Here's how the part is built. I have some questions about the finished solid (model axes, mm). Round coordinates to 2 decimals unless told otherwise and drop trailing zeros. Order: outer loops, then holes, each group sorted by start corner. A loop starts at its lowest first (then second) coordinate and runs counter-clockwise, first axis right, second up. Notation, with made-up numbers: (-0.75, -22.75) - (31.25, -22.75) arc R17 ccw to (31.25, -16.75) - close; hole circle Ø9 at (43, 6.25). An arc over 180 degrees is marked (long way). One line per item, written item: value.
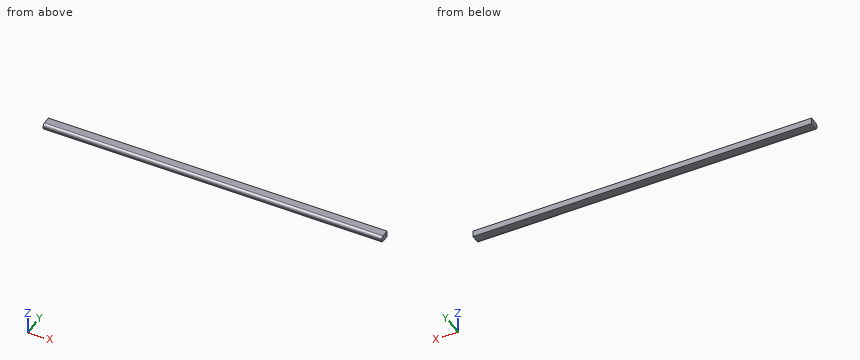
Autodesk Inventor part; units mm, degrees
ref_plane "YZ Plane" through (0, 0, 0) normal (1, 0, 0) x (0, 1, 0)
ref_plane "XZ Plane" through (0, 0, 0) normal (0, 1, 0) x (-1, 0, 0)
ref_plane "XY Plane" through (0, 0, 0) normal (0, 0, 1) x (1, 0, 0)
sketch "Sketch1" plane through (0, 0, 0) normal (0, 0, 1) x (1, 0, 0)
  line L0 (-592, 18) -> (592, 18)
  line L1 (592, 18) -> (592, -18)
  line L2 (592, -18) -> (-592, -18)
  line L3 (-592, -18) -> (-592, 18)
  line L4 (-592, 18) -> (592, -18) construction
  line L5 (592, 18) -> (-592, -18) construction
  point P0 (0, 0)
  dimension "d0" = 36
  dimension "d1" = 1184
extrude "Extrusion1" add sketch "Sketch1" along normal blind 22
fillet "Fillet1" radius 10 1 edges at (0, -18, 22)
fillet "Fillet2" radius 10 1 edges at (0, -18, 0)
properties part number "Light tube 118.4cm"
Q1. Will these pins go through, and if not, where does the flat tip stop? pin 1 (6 mm diameter, centred on x = -12, z = 5.5, fed in from -Y); pin 2 (6 mm diameter, centred on x = -54.5, z = 3, fed in from -Y); pin 3 (8 mm diameter, centred on x = -196.5, z = 19, fed in from -Y).
Results list:
pin 1: y = -17.89
pin 2: y = -17.17
pin 3: y = -17.54
Q2. If I drill on line 1 along Y through (x, z) = (-322, 13.5); line 2 along Y through (x, z) = (-509, 9.5); line 3 along Z through (x, y) = (472.5, -11), over which ranges is the centre line in solid material (lowest first)?
Results list:
line 1: -17.89 to 18
line 2: -17.99 to 18
line 3: 0.46 to 21.54
Q3. If we section it at B-B, the plane z = 15.5: Please give me the cut outline in (x, y), then the cut area to 3 significant figures.
Results list:
outline: (-592, -17.37) - (592, -17.37) - (592, 18) - (-592, 18) - close
area: 41,900 mm²
Q4. If we section it at A-A, the plane x = 476: Please give me the cut outline in (y, z).
Results list:
outline: (-18, 10) arc R10 ccw to (-8, 0) - (18, 0) - (18, 22) - (-8, 22) arc R10 ccw to (-18, 12) - close
